Design review of the part shown in the three views and the two pictorial views. Dimensions are in mm from the part's minimum x, y and z. A direction names the side the tool comes from. Give positions to 0.01 mm unless a question says otherwise; leave off trailing zeros. Order: outer loops, then holes, each group sorted by start corner. A loop starts at its lowest first (then second) coordinate and runs counter-clockwise, first axis right, second up.
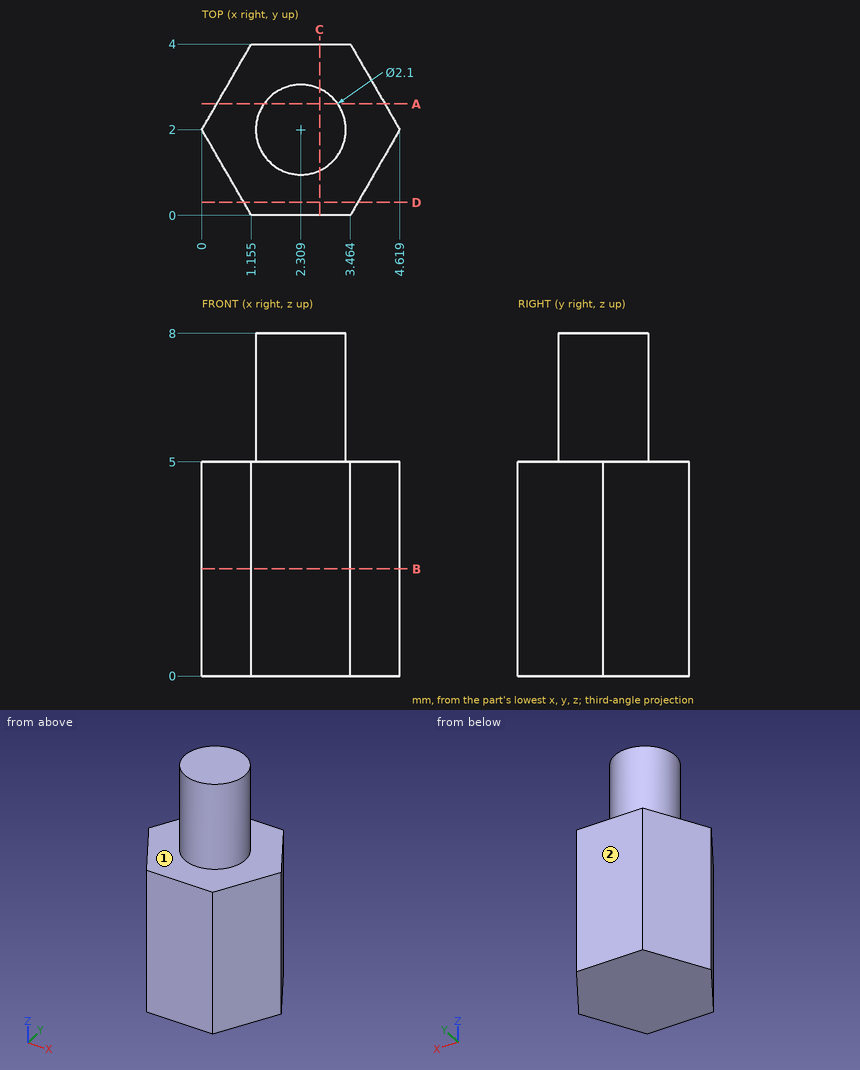
1) We need section C-C on x = 2.75. Give the boundary of the cut face in (y, z).
Answer sheet:
outline: (0, 0) - (4, 0) - (4, 5) - (2.95, 5) - (2.95, 8) - (1.05, 8) - (1.05, 5) - (0, 5) - close
2) We need section D-D on y = 0.3. Give the boundary of the cut face in (x, z).
Answer sheet:
outline: (0.98, 0) - (3.64, 0) - (3.64, 5) - (0.98, 5) - close
3) We need section B-B on z = 2.5. Give the boundary of the cut face in (x, y) (1 decimal).
Answer sheet:
outline: (0, 2) - (1.2, 0) - (3.5, 0) - (4.6, 2) - (3.5, 4) - (1.2, 4) - close
4) To check wall thickness, follow line 1 (Z direction, x = 3.35, y = 0.3); line 2 (X direction, y = 1.5, z = 3.75); line 3 (X direction, y = 3.05, z = 2) (1 decimal). State the ranges of each line that lie inside material, in increasing order.
Answer sheet:
line 1: z = 0 to 5
line 2: x = 0.29 to 4.33
line 3: x = 0.6 to 4
5) Clearance check with flat-ended pins moving along their axes: pin 1 (1.5 mm diameter, centred on x = 1, y = 3, fed in from -Z); pin 2 (1 mm diameter, centred on y = 0.5, z = 2.5, fed in from -X). State where each tip first meets the part, or that it passes through.
Answer sheet:
pin 1: stops at z = 0
pin 2: stops at x = 0.58
6) We need section A-A on y = 2.6. Give the boundary of the cut face in (x, z), then the cut area to 3 significant figures.
Answer sheet:
outline: (0.35, 0) - (4.27, 0) - (4.27, 5) - (3.17, 5) - (3.17, 8) - (1.45, 8) - (1.45, 5) - (0.35, 5) - close
area: 24.8 mm2
7) Tool access review of the marked faces 1 and 2: name each direction out of +Z, -Z, +X, -X, +Y, -Y from which nothing blocks a thin tool from reaching the whole face with its end or side.
Answer sheet:
face 1: +Z
face 2: +Z, -Z, +X, -X, +Y
